Can you work these out from the model? Positions are in its coordinate system, mm. Face numbers are marked on the shaded views. Give positions to 0.01 mm unless a question says otherwise; leave off trailing zeros. Order: outer loops, then holes, each group sorted by start corner. A loop starts at its lowest first (then second) coordinate and runs counter-clockwise, first axis right, second up.
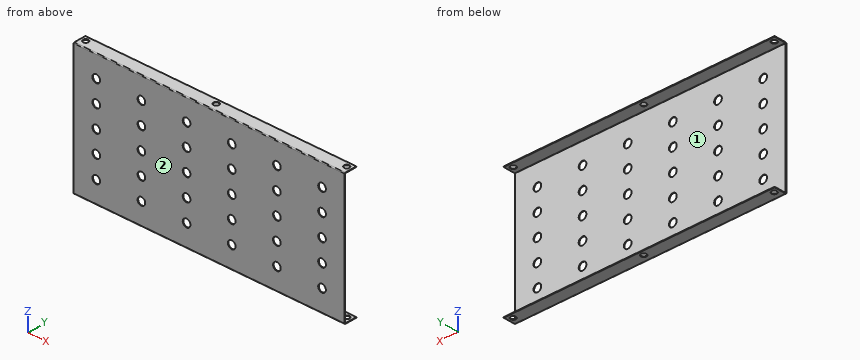
```python
from build123d import *

# Parameters (mm, degrees)
SKETCH_1_W                         = 300
SKETCH_1_H                         = 144
SKETCH_1_R                         = 4.25
SM_BASE_FLANGE_1_DEPTH             = 0.7
SM_EDGE_FLANGE_1_STRIP_W           = 3.2
SM_EDGE_FLANGE_1_STRIP_H           = 0.7
SM_EDGE_FLANGE_1_STRIP_CUT_DEPTH   = 300
SM_EDGE_FLANGE_1_STRIP_2_W         = 3.2
SM_EDGE_FLANGE_1_STRIP_2_H         = 0.7
SM_EDGE_FLANGE_1_STRIP_CUT_2_DEPTH = 300
SM_EDGE_FLANGE_1_DEPTH             = 300
SM_EDGE_FLANGE_1_BEND_DEPTH        = 300
SKETCH_14_R                        = 3
CUT_EXTRUDE_1_DEPTH                = 10
SKETCH_15_R                        = 3
CUT_EXTRUDE_2_DEPTH                = 10


# Sheet-metal steps are written as plain solids
with BuildPart() as part:
    # Sketch 1 → 基体-法兰1 (new body)
    with BuildSketch(Plane(origin=(0, 0, 0), x_dir=(1, 0, 0), z_dir=(0, 1, 0))):
        Rectangle(SKETCH_1_W, SKETCH_1_H)
        with Locations(Location((-125, -48, 0), (0, 0, 270))):
            Circle(SKETCH_1_R, mode=Mode.SUBTRACT)
        with Locations(Location((-125, -24, 0), (0, 0, 270))):
            Circle(SKETCH_1_R, mode=Mode.SUBTRACT)
        with Locations(Location((-125, 0, 0), (0, 0, 270))):
            Circle(SKETCH_1_R, mode=Mode.SUBTRACT)
        with Locations(Location((-125, 24, 0), (0, 0, 270))):
            Circle(SKETCH_1_R, mode=Mode.SUBTRACT)
        with Locations(Location((-125, 48, 0), (0, 0, 270))):
            Circle(SKETCH_1_R, mode=Mode.SUBTRACT)
        with Locations(Location((-75, -48, 0), (0, 0, 90))):
            Circle(SKETCH_1_R, mode=Mode.SUBTRACT)
        with Locations(Location((-75, -24, 0), (0, 0, 90))):
            Circle(SKETCH_1_R, mode=Mode.SUBTRACT)
        with Locations(Location((-75, 0, 0), (0, 0, 90))):
            Circle(SKETCH_1_R, mode=Mode.SUBTRACT)
        with Locations(Location((-75, 24, 0), (0, 0, 90))):
            Circle(SKETCH_1_R, mode=Mode.SUBTRACT)
        with Locations(Location((-75, 48, 0), (0, 0, 90))):
            Circle(SKETCH_1_R, mode=Mode.SUBTRACT)
        with Locations(Location((-25, -48, 0), (0, 0, 270))):
            Circle(SKETCH_1_R, mode=Mode.SUBTRACT)
        with Locations(Location((-25, -24, 0), (0, 0, 270))):
            Circle(SKETCH_1_R, mode=Mode.SUBTRACT)
        with Locations(Location((-25, 0, 0), (0, 0, 270))):
            Circle(SKETCH_1_R, mode=Mode.SUBTRACT)
        with Locations(Location((-25, 24, 0), (0, 0, 270))):
            Circle(SKETCH_1_R, mode=Mode.SUBTRACT)
        with Locations(Location((-25, 48, 0), (0, 0, 270))):
            Circle(SKETCH_1_R, mode=Mode.SUBTRACT)
        with Locations(Location((25, -48, 0), (0, 0, 90))):
            Circle(SKETCH_1_R, mode=Mode.SUBTRACT)
        with Locations(Location((25, -24, 0), (0, 0, 90))):
            Circle(SKETCH_1_R, mode=Mode.SUBTRACT)
        with Locations(Location((25, 0, 0), (0, 0, 90))):
            Circle(SKETCH_1_R, mode=Mode.SUBTRACT)
        with Locations(Location((25, 24, 0), (0, 0, 90))):
            Circle(SKETCH_1_R, mode=Mode.SUBTRACT)
        with Locations(Location((25, 48, 0), (0, 0, 90))):
            Circle(SKETCH_1_R, mode=Mode.SUBTRACT)
        with Locations(Location((75, 48, 0), (0, 0, 270))):
            Circle(SKETCH_1_R, mode=Mode.SUBTRACT)
        with Locations(Location((75, 24, 0), (0, 0, 270))):
            Circle(SKETCH_1_R, mode=Mode.SUBTRACT)
        with Locations(Location((75, 0, 0), (0, 0, 270))):
            Circle(SKETCH_1_R, mode=Mode.SUBTRACT)
        with Locations(Location((75, -24, 0), (0, 0, 270))):
            Circle(SKETCH_1_R, mode=Mode.SUBTRACT)
        with Locations(Location((75, -48, 0), (0, 0, 270))):
            Circle(SKETCH_1_R, mode=Mode.SUBTRACT)
        with Locations(Location((125, -48, 0), (0, 0, 90))):
            Circle(SKETCH_1_R, mode=Mode.SUBTRACT)
        with Locations(Location((125, -24, 0), (0, 0, 90))):
            Circle(SKETCH_1_R, mode=Mode.SUBTRACT)
        with Locations(Location((125, 0, 0), (0, 0, 90))):
            Circle(SKETCH_1_R, mode=Mode.SUBTRACT)
        with Locations(Location((125, 24, 0), (0, 0, 90))):
            Circle(SKETCH_1_R, mode=Mode.SUBTRACT)
        with Locations(Location((125, 48, 0), (0, 0, 90))):
            Circle(SKETCH_1_R, mode=Mode.SUBTRACT)
    extrude(amount=-SM_BASE_FLANGE_1_DEPTH)

    # 边线-法兰1 strip (across the edge) → 边线-法兰1 strip cut (cut)
    with BuildSketch(Plane(origin=(-150, 0, 72), x_dir=(0, 0, -1), z_dir=(1, 0, 0))):
        with Locations((-0.7, -0.35)):
            Rectangle(SM_EDGE_FLANGE_1_STRIP_W, SM_EDGE_FLANGE_1_STRIP_H)
    extrude(amount=SM_EDGE_FLANGE_1_STRIP_CUT_DEPTH, mode=Mode.SUBTRACT)

    # 边线-法兰1 strip 2 (across the edge) → 边线-法兰1 strip cut 2 (cut)
    with BuildSketch(Plane(origin=(150, 0, -72), x_dir=(0, 0, 1), z_dir=(-1, 0, 0))):
        with Locations((-0.7, -0.35)):
            Rectangle(SM_EDGE_FLANGE_1_STRIP_2_W, SM_EDGE_FLANGE_1_STRIP_2_H)
    extrude(amount=SM_EDGE_FLANGE_1_STRIP_CUT_2_DEPTH, mode=Mode.SUBTRACT)

    # 边线-法兰1 section (across the edge) → 边线-法兰1 (add)
    with BuildSketch(Plane(origin=(-150, 0, 72), x_dir=(0, 0, -1), z_dir=(1, 0, 0))):
        with BuildLine():
            Line((0, 0.2), (0, 13.3))
            Line((0, 13.3), (0.7, 13.3))
            Line((0.7, 13.3), (0.7, 0.2))
            ThreePointArc((0.7, 0.2), (0.758578644, 0.058578644), (0.9, 0))
            Line((0.9, 0), (0.9, -0.7))
            ThreePointArc((0.9, -0.7), (0.263603897, -0.436396103), (0, 0.2))
        make_face()
    extrude(amount=SM_EDGE_FLANGE_1_DEPTH)

    # 边线-法兰1 section 2 (across the edge) → 边线-法兰1 bend (add)
    with BuildSketch(Plane(origin=(150, 0, -72), x_dir=(0, 0, 1), z_dir=(-1, 0, 0))):
        with BuildLine():
            Line((0, 0.2), (0, 13.3))
            Line((0, 13.3), (0.7, 13.3))
            Line((0.7, 13.3), (0.7, 0.2))
            ThreePointArc((0.7, 0.2), (0.758578644, 0.058578644), (0.9, 0))
            Line((0.9, 0), (0.9, -0.7))
            ThreePointArc((0.9, -0.7), (0.263603897, -0.436396103), (0, 0.2))
        make_face()
    extrude(amount=SM_EDGE_FLANGE_1_BEND_DEPTH)

    # 草图14 → 切除-拉伸1 (cut)
    with BuildSketch(Plane(origin=(0, 0, 71.3), x_dir=(-1, 0, 0), z_dir=(0, 0, -1))):
        with Locations((-144.5, 7.8)):
            Circle(SKETCH_14_R)
        with Locations((0, 7.8)):
            Circle(SKETCH_14_R)
        with Locations((144.5, 7.8)):
            Circle(SKETCH_14_R)
    extrude(amount=-CUT_EXTRUDE_1_DEPTH, mode=Mode.SUBTRACT)

    # 草图15 → 切除-拉伸2 (cut)
    with BuildSketch(Plane(origin=(0, 0, -72), x_dir=(-1, 0, 0), z_dir=(0, 0, -1))):
        with Locations((-144.5, 7.8)):
            Circle(SKETCH_15_R)
        with Locations((0, 7.8)):
            Circle(SKETCH_15_R)
        with Locations((144.5, 7.8)):
            Circle(SKETCH_15_R)
    extrude(amount=-CUT_EXTRUDE_2_DEPTH, mode=Mode.SUBTRACT)


solid = part.part
```
1) Suppose I cut it at B-B (z = 48). Please give me the cut outline in (x, y), and give its area (3 significant figures).
2) We'd pull the mould along Z, two halves only. Please class the marked faces 1 and 2: +Z half, -Z half, draft (parallel to the pull), parting line (faces both ways), or undercut.
3) Suppose I cut it at A-A (x = -144.5). Please give me the cut outline in (y, z), and give its area (3 significant figures).
4) I'm going to push flat-ended pins straight in: pin 1 Ø7 at (x, z) = (-125, 0) entering from -Y; pin 2 Ø11 at (x, z) = (75, -24) entering from +Y. Where does each tip first touch, or does it pass through?
5) Suppose I cut it at C-C (y = 7.8). Give the number of separate pieces and of enclosed holes in the cut face, and give its area (3 significant figures).
6) If I drill on line 1 (Z direction, x = 62, y = 6.5); line 2 (Z direction, x = -75, y = -0.5); line 3 (Y direction, x = 48.5, z = -18), over which ranges is the centre line in solid material (lowest first)?
Results:
1. outline: (-150, -0.7) - (-129.25, -0.7) - (-129.25, 0) - (-150, 0) - close; (-120.75, -0.7) - (-79.25, -0.7) - (-79.25, 0) - (-120.75, 0) - close; (-70.75, -0.7) - (-29.25, -0.7) - (-29.25, 0) - (-70.75, 0) - close; (-20.75, -0.7) - (20.75, -0.7) - (20.75, 0) - (-20.75, 0) - close; (29.25, -0.7) - (70.75, -0.7) - (70.75, 0) - (29.25, 0) - close; (79.25, -0.7) - (120.75, -0.7) - (120.75, 0) - (79.25, 0) - close; (129.25, -0.7) - (150, -0.7) - (150, 0) - (129.25, 0) - close
1. area: 174 mm2
2. face 1: undercut
2. face 2: draft
3. outline: (-0.7, -71.1) arc R0.9 ccw to (0.2, -72) - (4.8, -72) - (4.8, -71.3) - (0.2, -71.3) arc R0.2 cw to (0, -71.1) - (0, 71.1) arc R0.2 cw to (0.2, 71.3) - (4.8, 71.3) - (4.8, 72) - (0.2, 72) arc R0.9 ccw to (-0.7, 71.1) - close; (10.8, -72) - (13.3, -72) - (13.3, -71.3) - (10.8, -71.3) - close; (10.8, 71.3) - (13.3, 71.3) - (13.3, 72) - (10.8, 72) - close
3. area: 111 mm2
4. pin 1: passes through
4. pin 2: stops at y = 0
5. separate pieces: 8
5. enclosed holes: 0
5. area: 395 mm2
6. line 1: z = -72 to -71.3, 71.3 to 72
6. line 2: z = -71.67 to -52.25, -43.75 to -28.25, -19.75 to -4.25, 4.25 to 19.75, 28.25 to 43.75, 52.25 to 71.67
6. line 3: y = -0.7 to 0
